from build123d import *

# Parameters (mm, degrees)
SKETCH_1_W               = 210
SKETCH_1_H               = 250
EXTRUDE_1_DEPTH          = 3
SKETCH_2_W               = 210
SKETCH_2_H               = 130
CUT_EXTRUDE_1_DEPTH      = 164.275840221
CUT_EXTRUDE_2_DEPTH      = 164.275840221
CUT_EXTRUDE_2_DEPTH_BACK = 164.275840221
SKETCH_4_W               = 20
SKETCH_4_H               = 60
FILLET_2_R               = 2
CUT_EXTRUDE_3_DEPTH      = 164.275840221
CUT_EXTRUDE_3_DEPTH_BACK = 164.275840221
SKETCH_7_R               = 1.6
SKETCH_7_R_2             = 1.55
SKETCH_8_R               = 1.6
SKETCH_8_R_2             = 1.5
CUT_EXTRUDE_4_DEPTH      = 164.275840221
SKETCH_9_W               = 210
SKETCH_9_H               = 90
EXTRUDE_2_DEPTH          = 3
SKETCH_10_R              = 2.1
CUT_EXTRUDE_5_DEPTH      = 10
SKETCH_11_R              = 1.25
CUT_EXTRUDE_6_DEPTH      = 240.288528768
SKETCH_12_R              = 2.1
CUT_EXTRUDE_7_DEPTH      = 10


with BuildPart() as part:
    # 草图1 → 凸台-拉伸1 (new body)
    with BuildSketch(Plane(origin=(0, 0, 0), x_dir=(1, 0, 0), z_dir=(0, 1, 0))):
        Rectangle(SKETCH_1_W, SKETCH_1_H)
    extrude(amount=EXTRUDE_1_DEPTH)

    # 草图2 → 切除-拉伸1 (cut, through all)
    with BuildSketch(Plane(origin=(0, 0, 0), x_dir=(1, 0, 0), z_dir=(0, 1, 0))):
        with Locations((0, -60)):
            Rectangle(SKETCH_2_W, SKETCH_2_H)
    extrude(amount=CUT_EXTRUDE_1_DEPTH, mode=Mode.SUBTRACT)

    # 草图4 → 切除-拉伸2 (cut, two sides: drawn at the far end of the back side and taken through both)
    with BuildSketch(Plane(origin=(0, 3, 0), x_dir=(1, 0, 0), z_dir=(0, 1, 0)).offset(-CUT_EXTRUDE_2_DEPTH_BACK)):
        with Locations((40, 65)):
            Rectangle(SKETCH_4_W, SKETCH_4_H)
    extrude(amount=CUT_EXTRUDE_2_DEPTH + CUT_EXTRUDE_2_DEPTH_BACK, mode=Mode.SUBTRACT)

    # 圆角2
    fillet_2_edges = [part.edges().sort_by_distance(p)[0] for p in [
        (50, 1.5, -95),
        (50, 1.5, -35),
        (30, 1.5, -35),
        (30, 1.5, -95),
    ]]
    fillet(fillet_2_edges, radius=FILLET_2_R)

    # 草图7 → 切除-拉伸3 (cut, two sides: drawn at the far end of the back side and taken through both)
    with BuildSketch(Plane(origin=(0, 3, 0), x_dir=(1, 0, 0), z_dir=(0, 1, 0)).offset(-CUT_EXTRUDE_3_DEPTH_BACK)):
        with Locations(Location((100, 120, 0), (0, 0, 270))):
            Circle(SKETCH_7_R)
        with Locations(Location((0, 120, 0), (0, 0, 270))):
            Circle(SKETCH_7_R_2)
        with Locations(Location((-100, 120, 0), (0, 0, 270))):
            Circle(SKETCH_7_R)
        with Locations(Location((-100, 10, 0), (0, 0, 270))):
            Circle(SKETCH_7_R)
        with Locations(Location((0, 10, 0), (0, 0, 270))):
            Circle(SKETCH_7_R_2)
        with Locations(Location((100, 10, 0), (0, 0, 270))):
            Circle(SKETCH_7_R)
    extrude(amount=CUT_EXTRUDE_3_DEPTH + CUT_EXTRUDE_3_DEPTH_BACK, mode=Mode.SUBTRACT)

    # 草图8 → 切除-拉伸4 (cut, through all)
    with BuildSketch(Plane(origin=(0, 3, 0), x_dir=(1, 0, 0), z_dir=(0, 1, 0))):
        with Locations(Location((20, 20, 0), (0, 0, 270))):
            Circle(SKETCH_8_R)
        with Locations(Location((-100, 20, 0), (0, 0, 270))):
            Circle(SKETCH_8_R)
        with Locations(Location((-100, 110, 0), (0, 0, 270))):
            Circle(SKETCH_8_R)
        with Locations(Location((20, 110, 0), (0, 0, 270))):
            Circle(SKETCH_8_R)
        with Locations(Location((-50, 10, 0), (0, 0, 270))):
            Circle(SKETCH_8_R_2)
        with Locations(Location((50, 10, 0), (0, 0, 90))):
            Circle(SKETCH_8_R_2)
        with Locations(Location((95, 26.4, 0), (0, 0, 270))):
            Circle(SKETCH_8_R)
        with Locations(Location((49.36, 26.4, 0), (0, 0, 270))):
            Circle(SKETCH_8_R)
        with Locations(Location((49.36, 103.6, 0), (0, 0, 270))):
            Circle(SKETCH_8_R)
        with Locations(Location((95, 103.6, 0), (0, 0, 270))):
            Circle(SKETCH_8_R)
    extrude(amount=-CUT_EXTRUDE_4_DEPTH, mode=Mode.SUBTRACT)

    # 草图9 → 凸台-拉伸2 (add)
    with BuildSketch(Plane(origin=(0, 3, 0), x_dir=(1, 0, 0), z_dir=(0, 1, 0))):
        with Locations((0, 170)):
            Rectangle(SKETCH_9_W, SKETCH_9_H)
    extrude(amount=-EXTRUDE_2_DEPTH)

    # 草图10 → 切除-拉伸5 (cut)
    with BuildSketch(Plane(origin=(0, 3, 0), x_dir=(1, 0, 0), z_dir=(0, 1, 0))):
        with Locations(Location((100, 132, 0), (0, 0, 270))):
            Circle(SKETCH_10_R)
        with Locations(Location((-100, 132, 0), (0, 0, 270))):
            Circle(SKETCH_10_R)
        with Locations(Location((0, 132, 0), (0, 0, 270))):
            Circle(SKETCH_10_R)
    extrude(amount=-CUT_EXTRUDE_5_DEPTH, mode=Mode.SUBTRACT)

    # 草图11 → 切除-拉伸6 (cut, through all)
    with BuildSketch(Plane(origin=(0, 0, 0), x_dir=(-1, 0, 0), z_dir=(0, -1, 0))):
        with Locations(Location((20, 210, 0), (0, 0, 90))):
            Circle(SKETCH_11_R)
        with Locations(Location((-20, 210, 0), (0, 0, 90))):
            Circle(SKETCH_11_R)
        with Locations(Location((28, 140.458645397, 0), (0, 0, 270))):
            Circle(SKETCH_11_R)
        with Locations(Location((-28, 140.458645397, 0), (0, 0, 90))):
            Circle(SKETCH_11_R)
    extrude(amount=-CUT_EXTRUDE_6_DEPTH, mode=Mode.SUBTRACT)

    # 草图12 → 切除-拉伸7 (cut)
    with BuildSketch(Plane(origin=(0, 3, 0), x_dir=(1, 0, 0), z_dir=(0, 1, 0))):
        with Locations(Location((100, 209, 0), (0, 0, 270))):
            Circle(SKETCH_12_R)
        with Locations(Location((-100, 209, 0), (0, 0, 270))):
            Circle(SKETCH_12_R)
    extrude(amount=-CUT_EXTRUDE_7_DEPTH, mode=Mode.SUBTRACT)


solid = part.part
Input: part model. Units: mm. Frame: model coordinates. Round coordinates to 2 decimals unless told otherwise and drop trailing zeros. Loops run counter-clockwise (first coordinate to the right, second up) from the corner with the lowest first, then second, coordinate; pieces in that order, holes last. Notation, with made-up numbers: (56, 58) -> (115, 58) arc R21 ccw to (115, 91) -> close; hole circle Ø11 at (82.25, 1.5). An arc over 180 degrees is marked (long way). Answer as a JSON object with one key per item and string values. Group by question number.
1) Section query A-A on z = -56.5. Output: boundary loops of the cut face in (x, y).
2) Ray query, L1, parallel to X at y = 1.5, z = -20; L2, parallel to X at y = 1.8, z = -40; L3, parallel to X at y = 1.75, z = -209. Return the intervals inside material, ascending.
3) Section query B-B on y = 1.4. State how many separate pieces and enclosed holes the cut face has, plus the area to 3 significant figures.
Reply:
{
 "1": {"outline": "(-105, 0) -> (30, 0) -> (30, 3) -> (-105, 3) -> close; (50, 0) -> (105, 0) -> (105, 3) -> (50, 3) -> close"},
 "2": {"L1": "x = -105 to -101.6, -98.4 to 18.4, 21.6 to 105", "L2": "x = -105 to 30, 50 to 105", "L3": "x = -105 to -102.1, -97.9 to -20.75, -19.25 to 19.25, 20.75 to 97.9, 102.1 to 105"},
 "3": {"separate pieces": "1", "enclosed holes": "26", "area": "42,700 mm2"}
}
